Input: part model. Units: mm. Frame: model coordinates. A direction names the side the tool comes from. Coordinates: 2 decimals unless noted, no trailing zeros. Loops run counter-clockwise (first coordinate to the right, second up) from the corner with the lowest first, then second, coordinate; pieces in that order, holes last.
(1) Line query: L1, parallel to Z at x = 21.5, y = -1.6 (3 decimals); L2, parallel to Z at x = 73, y = -1.6 (3 decimals); L3, parallel to X at y = -0.25, z = 52 (3 decimals). Output: solid intervals per line, ascending.
(2) Section D-D, the plane z = -39.2. Return loops of the section in (x, y) (3 decimals).
(3) Section A-A, the plane z = -77.7. Return loops of the section in (x, y) (3 decimals), then the cut area to 3 significant figures.
(4) Set-up query: faces 4 (the face through (99.496, -1.61, -39.589)), 5 (the face through (102.96, -1.57, 96.52)). Return all of +Z, -Z, +X, -X, +Y, -Y with unobstructed straight access to the full face (end or side cutting, diameter ignored); none if empty.
(5) Section C-C, the plane y = -0.9. Return loops of the section in (x, z) (3 decimals).
(6) Mould query, pull axis Z, two halves, no side actions, for faces 1 (the face through (3.226, -1.61, -72.641)), 2 (the face through (-102.87, -1.57, 96.61)), 3 (the face through (-102.96, -1.57, -96.52)). Classes: released by +Z, released by -Z, zero draft, split by the parting line, or undercut.
(7) Section B-B, the plane x = 37. Return loops of the section in (y, z) (3 decimals), then the cut area to 3 significant figures.
```python
from build123d import *

# Parameters (mm, degrees)
F1_DEPTH = 3.175
F2_R     = 3.175
F3_DEPTH = 25.4
F5_DEPTH = 25
F6_DEPTH = 25
F7_DEPTH = 25
F8_R     = 6
F9_DEPTH = 25


with BuildPart() as f1:
    # F0 (on Front) → F1 (new body)
    with BuildSketch(Plane.XZ):
        with BuildLine():
            Line((98.425, 98.425), (-98.425, 98.425))
            ThreePointArc((-98.425, 98.425), (-102.915128, 96.565128), (-104.775, 92.075))
            Line((-104.775, 92.075), (-104.775, -92.075))
            ThreePointArc((-104.775, -92.075), (-102.915128, -96.565128), (-98.425, -98.425))
            Line((-98.425, -98.425), (98.425, -98.425))
            ThreePointArc((98.425, -98.425), (102.915128, -96.565128), (104.775, -92.075))
            Line((104.775, -92.075), (104.775, 92.075))
            ThreePointArc((104.775, 92.075), (102.915128, 96.565128), (98.425, 98.425))
        make_face()
    extrude(amount=F1_DEPTH)

    # F2 (on face) → F3 (cut)
    with BuildSketch(Plane.XZ.offset(3.175)):
        with Locations((-98.425, 92.075)):
            Circle(F2_R)
        with Locations((98.425, 92.075)):
            Circle(F2_R)
        with Locations((98.425, -92.075)):
            Circle(F2_R)
        with Locations((-98.425, -92.075)):
            Circle(F2_R)
    extrude(amount=-F3_DEPTH, mode=Mode.SUBTRACT)

    # F4 (on face) → F5 (cut)
    with BuildSketch(Plane.XZ.offset(3.175)):
        with BuildLine():
            ThreePointArc((-65, 78.4), (-99.5, 43.9), (-65, 9.4))
            Line((-65, 9.4), (65, 9.4))
            ThreePointArc((65, 9.4), (99.5, 43.9), (65, 78.4))
            Line((65, 78.4), (-65, 78.4))
        make_face()
        with BuildLine():
            ThreePointArc((-81.8, -21.5), (-99.5, -39.2), (-81.8, -56.9))
            Line((-81.8, -56.9), (81.8, -56.9))
            ThreePointArc((81.8, -56.9), (99.5, -39.2), (81.8, -21.5))
            Line((81.8, -21.5), (-81.8, -21.5))
        make_face()
    extrude(amount=-F5_DEPTH, mode=Mode.SUBTRACT)

    # F4 (on face) → F6 (cut)
    with BuildSketch(Plane.XZ.offset(3.175)):
        with BuildLine():
            ThreePointArc((-65, 78.4), (-99.5, 43.9), (-65, 9.4))
            Line((-65, 9.4), (65, 9.4))
            ThreePointArc((65, 9.4), (99.5, 43.9), (65, 78.4))
            Line((65, 78.4), (-65, 78.4))
        make_face()
        with BuildLine():
            ThreePointArc((-81.8, -21.5), (-99.5, -39.2), (-81.8, -56.9))
            Line((-81.8, -56.9), (81.8, -56.9))
            ThreePointArc((81.8, -56.9), (99.5, -39.2), (81.8, -21.5))
            Line((81.8, -21.5), (-81.8, -21.5))
        make_face()
    extrude(amount=-F6_DEPTH, mode=Mode.SUBTRACT)

    # F4 (on face) → F7 (cut)
    with BuildSketch(Plane.XZ.offset(3.175)):
        with BuildLine():
            ThreePointArc((-65, 78.4), (-99.5, 43.9), (-65, 9.4))
            Line((-65, 9.4), (65, 9.4))
            ThreePointArc((65, 9.4), (99.5, 43.9), (65, 78.4))
            Line((65, 78.4), (-65, 78.4))
        make_face()
        with BuildLine():
            ThreePointArc((-81.8, -21.5), (-99.5, -39.2), (-81.8, -56.9))
            Line((-81.8, -56.9), (81.8, -56.9))
            ThreePointArc((81.8, -56.9), (99.5, -39.2), (81.8, -21.5))
            Line((81.8, -21.5), (-81.8, -21.5))
        make_face()
    extrude(amount=-F7_DEPTH, mode=Mode.SUBTRACT)

    # F8 (on face) → F9 (cut)
    with BuildSketch(Plane.XZ.offset(3.175)):
        with Locations((0, -77.7)):
            Circle(F8_R)
    extrude(amount=-F9_DEPTH, mode=Mode.SUBTRACT)


solid = f1.part
```
Report:
1. L1: z = -98.425 to -56.9, -21.5 to 9.4, 78.4 to 98.425
1. L2: z = -98.425 to -56.9, -21.5 to 10.34, 77.46 to 98.425
1. L3: x = -104.775 to -98.536, 98.536 to 104.775
2. outline: (-104.775, -3.175) - (-99.5, -3.175) - (-99.5, 0) - (-104.775, 0) - close; (99.5, -3.175) - (104.775, -3.175) - (104.775, 0) - (99.5, 0) - close
3. outline: (-104.775, -3.175) - (-6, -3.175) - (-6, 0) - (-104.775, 0) - close; (6, -3.175) - (104.775, -3.175) - (104.775, 0) - (6, 0) - close
3. area: 627 mm2
4. face 4: +Y, -Y
4. face 5: +Z, +X, +Y, -Y
5. outline: (-104.775, -92.075) arc R6.35 ccw to (-98.425, -98.425) - (98.425, -98.425) arc R6.35 ccw to (104.775, -92.075) - (104.775, 92.075) arc R6.35 ccw to (98.425, 98.425) - (-98.425, 98.425) arc R6.35 ccw to (-104.775, 92.075) - close; hole circle Ø6.35 at (-98.425, -92.075); hole circle Ø6.35 at (-98.425, 92.075); hole (-81.8, -56.9) - (81.8, -56.9) arc R17.7 ccw to (81.8, -21.5) - (-81.8, -21.5) arc R17.7 ccw to start; hole (-65, 9.4) - (65, 9.4) arc R34.5 ccw to (65, 78.4) - (-65, 78.4) arc R34.5 ccw to start; hole circle Ø12 at (0, -77.7); hole circle Ø6.35 at (98.425, -92.075); hole circle Ø6.35 at (98.425, 92.075)
6. face 1: undercut
6. face 2: released by +Z
6. face 3: released by -Z
7. outline: (-3.175, -98.425) - (0, -98.425) - (0, -56.9) - (-3.175, -56.9) - close; (-3.175, -21.5) - (0, -21.5) - (0, 9.4) - (-3.175, 9.4) - close; (-3.175, 78.4) - (0, 78.4) - (0, 98.425) - (-3.175, 98.425) - close
7. area: 294 mm2
